Check sheet for the drawn part. Datum: minimum x, y, z corner. Units: mm. Coordinates: 2 decimals unless noted, no trailing zeros. Write each loop counter-clockwise with the first axis right and the second up, starting at its lowest first coordinate (ties: lowest second). Pieces come first, ordered by that corner, then holes. Notation, with made-up numbers: (24, 87.5) -> (44, 87.5) arc R30 ccw to (44, 114.5) -> close; hole circle Ø4 at (-2, -34.5). An arc over 180 degrees is marked (long way). Write item = value, one per line. Start each with the question number.
(1) Material ranges on probe 1 along Z at (x, y) = (6, 7.5); probe 2 along X at (y, z) = (8, 16.5); probe 3 along X at (y, z) = (7, 27), recorded low to high. Write a range as [from, to].
(2) Section check C-C (z = 26.5). Record the cut outline in (x, y), plus the area to 3 significant figures.
(3) Section check B-B (x = 51). Record the cut outline in (y, z).
(4) Mould release check, pull along Z, two halves, no side actions. Record for the marked faces 1, 2 and 3: released by +Z, released by -Z, zero draft, split by the parting line, or undercut.
(5) Section check A-A (z = 16.5). Record the cut outline in (x, y).
(6) Section check D-D (y = 8.25). Record the cut outline in (x, z).
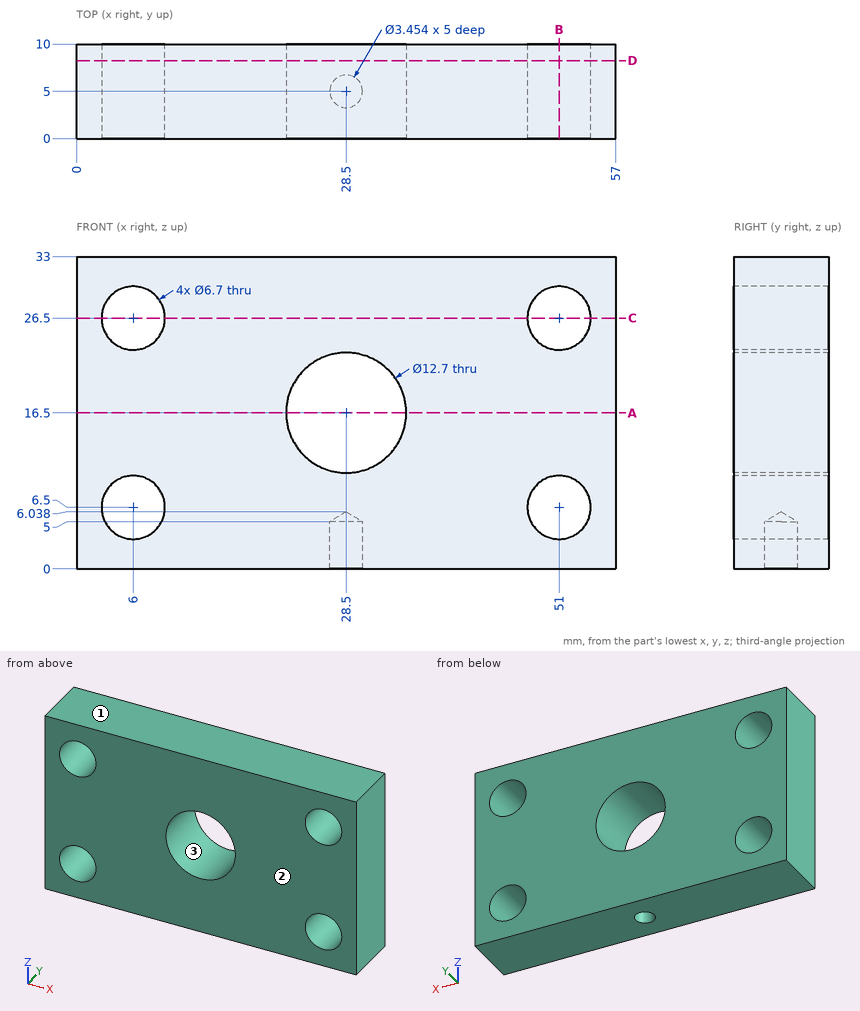
Response:
q1.probe_1 = [0, 3.15], [9.85, 23.15], [29.85, 33]
q1.probe_2 = [0, 22.15], [34.85, 57]
q1.probe_3 = [0, 2.69], [9.31, 47.69], [54.31, 57]
q2.outline = (0, 0) -> (2.65, 0) -> (2.65, 10) -> (0, 10) -> close; (9.35, 0) -> (47.65, 0) -> (47.65, 10) -> (9.35, 10) -> close; (54.35, 0) -> (57, 0) -> (57, 10) -> (54.35, 10) -> close
q2.area = 436 mm2
q3.outline = (0, 0) -> (10, 0) -> (10, 3.15) -> (0, 3.15) -> close; (0, 9.85) -> (10, 9.85) -> (10, 23.15) -> (0, 23.15) -> close; (0, 29.85) -> (10, 29.85) -> (10, 33) -> (0, 33) -> close
q4.face_1 = released by +Z
q4.face_2 = zero draft
q4.face_3 = undercut
q5.outline = (0, 0) -> (22.15, 0) -> (22.15, 10) -> (0, 10) -> close; (34.85, 0) -> (57, 0) -> (57, 10) -> (34.85, 10) -> close
q6.outline = (0, 0) -> (57, 0) -> (57, 33) -> (0, 33) -> close; hole circle Ø6.7 at (6, 6.5); hole circle Ø6.7 at (6, 26.5); hole circle Ø12.7 at (28.5, 16.5); hole circle Ø6.7 at (51, 6.5); hole circle Ø6.7 at (51, 26.5)
